Work out the finished part from the listing and answer in its coordinate system (mm). A direction names the side the tool comes from. Round coordinates to 2 decimals unless told otherwise and drop trailing zeros. Order: outer loops, then holes, each group sorted by start corner. A loop starts at its lowest first (then second) coordinate and runs counter-clockwise, first axis right, second up. Notation, with made-up numbers: M 42,57 L 58,57 A31 ccw 58,96 Z; hole C -27.75,22 d4. An arc over 180 degrees is marked long. Answer as a JSON object with one key per item and string values. Group by question number.
Autodesk Inventor part; units mm, degrees
ref_plane "YZ Plane" through (0, 0, 0) normal (1, 0, 0) x (0, 1, 0)
ref_plane "XZ Plane" through (0, 0, 0) normal (0, 1, 0) x (-1, 0, 0)
ref_plane "XY Plane" through (0, 0, 0) normal (0, 0, 1) x (1, 0, 0)
sketch "Sketch1" plane through (0, 0, 0) normal (0, 1, 0) x (-1, 0, 0)
  circle A0 centre (0, 0) radius 5
  dimension "d0" = 10
extrude "Extrusion1" add sketch "Sketch1" along normal blind 3.1
chamfer "Chamfer1" distance 3.1 angle 45 1 edges at (5, 0, 0)
sketch "Sketch2" plane through (0, 0, 0) normal (0, -1, 0) x (1, 0, 0)
  circle A0 centre (0, 0) radius 1.9
  circle A1 centre (0, 0) radius 2.5
  dimension "d7" = 5
extrude "Extrusion2" add sketch "Sketch2" along normal blind 6.9 and the other way blind 1 contours A0 | A1
chamfer "Chamfer2" distance 0.5 angle 45 1 edges at (-2.5, -6.9, 0)
sketch "Sketch3" plane through (0, 3.1, 0) normal (0, 1, 0) x (1, 0, 0)
  circle A0 centre (0, 0) radius 5
  line L0 (0, 1.7321) -> (1.5, 0.866)
  line L1 (1.5, 0.866) -> (1.5, -0.866)
  line L2 (1.5, -0.866) -> (0, -1.7321)
  line L3 (0, -1.7321) -> (-1.5, -0.866)
  line L4 (-1.5, -0.866) -> (-1.5, 0.866)
  line L5 (-1.5, 0.866) -> (0, 1.7321)
  dimension "d15" = 3
extrude "Extrusion3" cut sketch "Sketch3" against normal blind 2 contours L0 L1 L2 L3 L4 L5
thread "Thread1"
properties part number "M5x10FHS"
Item 1: Each of these flat-tipped pins is pushed along its axis until it touches: pin 1 (5 mm diameter, centred on y = 1.5, z = 0.5, fed in from -X); pin 2 (0.9 mm diameter, centred on x = -0.5, z = 0.5, fed in from +Y); pin 3 (4 mm diameter, centred on y = -3, z = -1, fed in from -X); pin 4 (0.9 mm diameter, centred on y = 2, z = 0, fed in from -X). Where does it stop, or does it pass through?
Item 2: Find section A-A (y = -4.5). Give the vertices of the cut face in (x, z), and give its area (3 significant figures).
Item 3: Consider L1, parallel to Z at x = 2, y = -4.75; L2, parallel to Y at x = -0.75, z = 1.25; L3, parallel to X at y = -3.5, z = -1.5. Determine where each line is inside the solid, lowest interval first.
Item 4: The mould has two halves that part along Z. Classify faces 3 (the flat face through (0.74, 2.114, -1.305)), 4 (the cylindrical face through (-0.54, -2.95, -2.44)), 5 (the flat face through (-0.74, 2.114, 1.305)), 6 (the flat face through (0, -6.9, 0)): +Z half, -Z half, draft (parallel to the pull), parting line (faces both ways), or undercut.
Item 5: A tool of negligible diameter and unlimited length cuts with its end or side. For faces 1 (the flat face through (-2, 3.1, 0)), 2 (the flat face through (0.76, 2.114, 1.293)), from which of +Z, -Z, +X, -X, +Y, -Y can it reach the whole face along a straight path? Write none if from no direction.
Responses:
{
 "1": {"pin 1": "stops at x = -5", "pin 2": "stops at y = 1.1", "pin 3": "stops at x = -2.5", "pin 4": "stops at x = -4.35"},
 "2": {"outline": "C 0,0 d5", "area": "19.6 mm^2"},
 "3": {"L1": "z = -1.5 to 1.5", "L2": "y = -6.9 to 1.1", "L3": "x = -2 to 2"},
 "4": {"face 3": "undercut", "face 4": "parting line", "face 5": "undercut", "face 6": "draft"},
 "5": {"face 1": "+Z, -Z, +X, -X, +Y", "face 2": "+Y"}
}
